The figure shows three views and two pictorial views of one solid part (mm, origin at its lowest corner). Answer the questions. A direction names the side the tool comes from. Give positions to 0.01 mm unless a question says otherwise; leave off trailing zeros. Loops run counter-clockwise (first coordinate to the right, second up) from the corner with the lowest first, then second, coordinate; pieces in that order, holes last. Notation, with made-up numbers: (33.5, -12) -> (44.5, -12) arc R27 cw to (44.5, 23) -> close; hole circle Ø1 at (38, -20.75). An arc over 180 degrees is marked (long way). Answer as CSV lines item,"result". Start each with the question number.
1. Find the intervals of material crossed by line 1 along Z through (x, y) = (6.75, 6.35) (1 decimal); line 2 along Y through (x, z) = (10, 30); line 3 along Z through (x, y) = (11.25, 21), in increasing order.
2. Find section A-A, the plane y = 6.35. Give the vertices of the cut face in (x, z) (1 decimal).
3. Find section C-C, the plane z = 25.5. Give the vertices of the cut face in (x, y), and give its area (3 significant figures).
4. Flat-ended cylindrical pins translate along their axes: pin 1 Ø6 at (x, z) = (5, 63.5) entering from +Y; pin 2 Ø10 at (y, z) = (6.35, 63.69) entering from +X; pin 3 Ø6.5 at (x, y) = (5.5, 33) entering from -Z. Find the tip coordinate at first contact, or state that the pin passes through.
5. Find section D-D, the plane y = 42.5. Give the vertices of the cut face in (x, z).
6. Find section B-B, the plane x = 6. Count the separate pieces of the cut face and the enclosed holes in it, and give its area (3 significant figures).
7. A tool of negligible diameter and unlimited length cuts with its end or side. For the marked faces 1 and 2, from which of +Z, -Z, +X, -X, +Y, -Y can it reach the whole face along a straight path? Write none if from no direction.
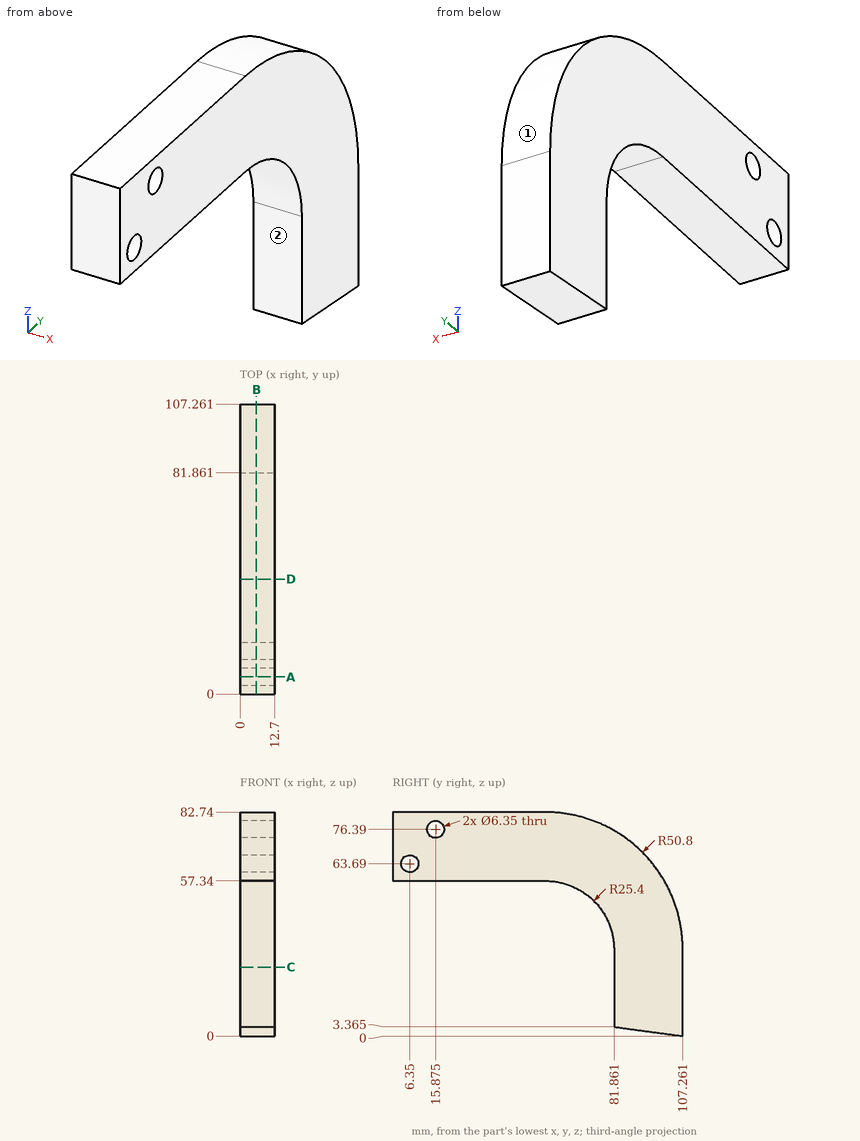
Resolved:
1,line 1,"z = 57.3 to 60.5, 66.9 to 82.7"
1,line 2,"y = 81.86 to 107.26"
1,line 3,"z = 57.34 to 82.74"
2,outline,"(0, 57.3) -> (12.7, 57.3) -> (12.7, 60.5) -> (0, 60.5) -> close; (0, 66.9) -> (12.7, 66.9) -> (12.7, 82.7) -> (0, 82.7) -> close"
3,outline,"(0, 81.86) -> (12.7, 81.86) -> (12.7, 107.26) -> (0, 107.26) -> close"
3,area,"323 mm^2"
4,pin 1,"stops at y = 98.47"
4,pin 2,"stops at x = 12.7"
4,pin 3,"stops at z = 57.34"
5,outline,"(0, 57.34) -> (12.7, 57.34) -> (12.7, 82.74) -> (0, 82.74) -> close"
6,separate pieces,"1"
6,enclosed holes,"2"
6,area,"3,660 mm^2"
7,face 1,"+Z, +X, -X, +Y"
7,face 2,"-Z, +X, -X, -Y"
